Verification items for the finished model (mm, model axes). A direction names the side the tool comes from. Coordinates: 2 decimals unless noted, no trailing zeros. Write each loop counter-clockwise with the first axis right and the second up, starting at its lowest first coordinate (ties: lowest second). Pieces come first, ordered by that corner, then holes. Notation, with made-up numbers: (-35, 11.25) - (-30, 11.25) arc R21 ccw to (-30, 36.25) - close; hole circle Ø10 at (13.25, 25.5). An arc over 180 degrees is marked (long way). Use one line per item in the form item = value. Start each with the question number.
(1) Sectioned sample at A-A (z = 4.8). Record the cut outline in (x, y), and give its area (4 significant figures).
(2) Material ranges on line 1 (Z direction, x = 59.5, y = 18); line 2 (X direction, y = 38.5, z = 4.8); line 3 (Z direction, x = 56.7, y = 39.55), recorded low to high. Write a range as [from, to].
(3) Tool access check on faces 1 (the cylindrical face through (9.9, 11.3, -2.8)), 2 (the cylindrical face through (53.6, 39.53, 7.93)), 3 (the flat face through (44.376, -0.74, 59.833)). Record the directions out of +Z, -Z, +X, -X, +Y, -Y that give a thin tool (end or side, any length) a straight path to the whole face; none if there is none.
(4) Sectioned sample at D-D (z = 49). Record the cut outline in (x, y).
(5) Sectioned sample at B-B (y = 30.5). Record the cut outline in (x, z).
(6) Gauge pin test, flat ends, axial feed: pin 1 Ø2.5 at (x, z) = (58.5, 11.5) entering from +Y; pin 2 Ø4 at (x, y) = (52, 33) entering from -Z. Record the tip position at first contact, or that the pin passes through.
(7) Sectioned sample at C-C (z = 73.2). Count the separate pieces of the cut face and the enclosed holes in it, and give its area (3 significant figures).
(8) Mould release check, pull along Z, two halves, no side actions. Record for faces 4 (the flat face through (3, 37, 75)), 5 (the flat face through (-0.5, 42, 47.8)): released by +Z, released by -Z, zero draft, split by the parting line, or undercut.
from build123d import *

# Parameters (mm, degrees)
ESBO_O1_W                 = 63
ESBO_O1_H                 = 45
ESBO_O1_W_2               = 60
ESBO_O1_H_2               = 42
RESSALTO_EXTRUS_O2_DEPTH  = 1.5
RESSALTO_EXTRUS_O3_START  = 1.5
ESBO_O1_3_W               = 63
ESBO_O1_3_H               = 45
ESBO_O1_3_W_2             = 60
ESBO_O1_3_H_2             = 42
RESSALTO_EXTRUS_O3_DEPTH  = 75
RESSALTO_EXTRUS_O4_DEPTH  = 15
CORTE_EXTRUS_O1_DEPTH     = 27
ESBO_O4_W                 = 63
ESBO_O4_H                 = 45
RESSALTO_EXTRUS_O6_DEPTH  = 1.5
ESBO_O5_W                 = 63
ESBO_O5_H                 = 1.5
CORTE_EXTRUS_O2_DEPTH     = 109.436617432
RESSALTO_EXTRUS_O7_START  = 42
ESBO_O6_R                 = 1.3
RESSALTO_EXTRUS_O7_DEPTH  = 5
ESPELHAR2_START           = 42
ESPELHAR2_COPY_1_SKETCH_R = 1.3
ESPELHAR2_COPY_1_DEPTH    = 5
RESSALTO_EXTRUS_O8_START  = -5.5
RESSALTO_EXTRUS_O8_DEPTH  = 5.5
ESBO_O7_W                 = 3
ESBO_O7_H                 = 3
RESSALTO_EXTRUS_O9_DEPTH  = 25.5


with BuildPart() as part:
    # Esboço1 → Ressalto-extrusão2 (new body)
    # profile 1 of 3: a face of its own
    with BuildSketch(Plane.XY):
        with Locations((30, 21)):
            Rectangle(ESBO_O1_W, ESBO_O1_H)
        with Locations((30, 21)):
            Rectangle(ESBO_O1_W_2, ESBO_O1_H_2, mode=Mode.SUBTRACT)
    # profile 2 of 3: a face of its own
    with BuildSketch(Plane.XY):
        with Locations((30, 21)):
            Rectangle(ESBO_O1_W_2, ESBO_O1_H_2)
        with BuildLine():
            ThreePointArc((12.174114264, 11.987815308), (11.9, 11.3), (12.174114264, 10.612184692))
            Line((12.174114264, 10.612184692), (18.25, 4.2))
            Line((18.25, 4.2), (41.75, 4.2))
            Line((41.75, 4.2), (47.825885736, 10.612184692))
            ThreePointArc((47.825885736, 10.612184692), (48.1, 11.3), (47.825885736, 11.987815308))
            Line((47.825885736, 11.987815308), (41.75, 18.4))
            Line((41.75, 18.4), (18.25, 18.4))
            Line((18.25, 18.4), (12.174114264, 11.987815308))
        make_face(mode=Mode.SUBTRACT)
    # profile 3 of 3: a face of its own
    with BuildSketch(Plane.XY):
        with Locations((30, 21)):
            Rectangle(ESBO_O1_W_2, ESBO_O1_H_2)
        with BuildLine():
            ThreePointArc((10.722342792, 13.363445925), (9.9, 11.3), (10.722342792, 9.236554075))
            Line((10.722342792, 9.236554075), (17.389851698, 2.2))
            Line((17.389851698, 2.2), (42.610148302, 2.2))
            Line((42.610148302, 2.2), (49.277657208, 9.236554075))
            ThreePointArc((49.277657208, 9.236554075), (50.1, 11.3), (49.277657208, 13.363445925))
            Line((49.277657208, 13.363445925), (42.610148302, 20.4))
            Line((42.610148302, 20.4), (17.389851698, 20.4))
            Line((17.389851698, 20.4), (10.722342792, 13.363445925))
        make_face(mode=Mode.SUBTRACT)
    extrude(amount=RESSALTO_EXTRUS_O2_DEPTH)

    # Esboço1<3> → Ressalto-extrusão3 (add)
    with BuildSketch(Plane.XY.offset(RESSALTO_EXTRUS_O3_START)):
        with Locations((30, 21)):
            Rectangle(ESBO_O1_3_W, ESBO_O1_3_H)
        with Locations((30, 21)):
            Rectangle(ESBO_O1_3_W_2, ESBO_O1_3_H_2, mode=Mode.SUBTRACT)
    extrude(amount=RESSALTO_EXTRUS_O3_DEPTH)

    # Esboço2 → Ressalto-extrusão4 (add)
    with BuildSketch(Plane(origin=(0, 0, 0), x_dir=(1, 0, 0), z_dir=(0, 1, 0))):
        with BuildLine():
            Line((18.25, -54.8), (41.75, -54.8))
            Line((41.75, -54.8), (48.66440786, -62.248218844))
            ThreePointArc((48.66440786, -62.248218844), (49.654140055, -63.822712297), (50, -65.65))
            Line((50, -65.65), (51.5, -65.65))
            ThreePointArc((51.5, -65.65), (51.050382071, -63.274525986), (49.763730218, -61.227684497))
            Line((49.763730218, -61.227684497), (42.404219824, -53.3))
            Line((42.404219824, -53.3), (17.595780176, -53.3))
            Line((17.595780176, -53.3), (10.236269782, -61.227684497))
            ThreePointArc((10.236269782, -61.227684497), (8.949617929, -63.274525986), (8.5, -65.65))
            Line((8.5, -65.65), (10, -65.65))
            ThreePointArc((10, -65.65), (10.345859945, -63.822712297), (11.33559214, -62.248218844))
            Line((11.33559214, -62.248218844), (18.25, -54.8))
        make_face()
        with BuildLine():
            ThreePointArc((11.33559214, -69.051781156), (10.345859945, -67.477287703), (10, -65.65))
            Line((10, -65.65), (8.5, -65.65))
            ThreePointArc((8.5, -65.65), (8.949617929, -68.025474014), (10.236269782, -70.072315503))
            Line((10.236269782, -70.072315503), (16.2032846, -76.5))
            Line((16.2032846, -76.5), (18.25, -76.5))
            Line((18.25, -76.5), (11.33559214, -69.051781156))
        make_face()
        with BuildLine():
            Line((51.5, -65.65), (50, -65.65))
            ThreePointArc((50, -65.65), (49.654140055, -67.477287703), (48.66440786, -69.051781156))
            Line((48.66440786, -69.051781156), (41.75, -76.5))
            Line((41.75, -76.5), (43.7967154, -76.5))
            Line((43.7967154, -76.5), (49.763730218, -70.072315503))
            ThreePointArc((49.763730218, -70.072315503), (51.050382071, -68.025474014), (51.5, -65.65))
        make_face()
    extrude(amount=RESSALTO_EXTRUS_O4_DEPTH)

    # Esboço2<3> → Corte-extrusão1 (cut)
    with BuildSketch(Plane(origin=(0, 0, 0), x_dir=(1, 0, 0), z_dir=(0, 1, 0))):
        with BuildLine():
            Line((41.095780176, -56.3), (30, -56.3))
            Line((30, -56.3), (30, -75))
            Line((30, -75), (41.095780176, -75))
            Line((41.095780176, -75), (47.565085502, -68.031246809))
            ThreePointArc((47.565085502, -68.031246809), (48.5, -65.65), (47.565085502, -63.268753191))
            Line((47.565085502, -63.268753191), (41.095780176, -56.3))
        make_face()
        with BuildLine():
            Line((30, -75), (30, -56.3))
            Line((30, -56.3), (18.904219824, -56.3))
            Line((18.904219824, -56.3), (12.434914498, -63.268753191))
            ThreePointArc((12.434914498, -63.268753191), (11.5, -65.65), (12.434914498, -68.031246809))
            Line((12.434914498, -68.031246809), (18.904219824, -75))
            Line((18.904219824, -75), (30, -75))
        make_face()
    extrude(amount=-CORTE_EXTRUS_O1_DEPTH, mode=Mode.SUBTRACT)

    # Esboço4 → Ressalto-extrusão6 (add)
    with BuildSketch(Plane.XY.offset(76.5)):
        with Locations((30, 21)):
            Rectangle(ESBO_O4_W, ESBO_O4_H)
    extrude(amount=RESSALTO_EXTRUS_O6_DEPTH)

    # Esboço5 → Corte-extrusão2 (cut, through all)
    with BuildSketch(Plane.XY.offset(78)):
        with Locations((30, 42.75)):
            Rectangle(ESBO_O5_W, ESBO_O5_H)
    extrude(amount=-CORTE_EXTRUS_O2_DEPTH, mode=Mode.SUBTRACT)

    # Esboço6 → Ressalto-extrusão7 (add)
    with BuildSketch(Plane(origin=(0, 0, 0), x_dir=(1, 0, 0), z_dir=(0, 1, 0)).offset(RESSALTO_EXTRUS_O7_START)):
        with BuildLine():
            Line((60, -1.5), (60, -8.5))
            Line((60, -8.5), (55, -8.5))
            ThreePointArc((55, -8.5), (53.585786438, -7.914213562), (53, -6.5))
            Line((53, -6.5), (53, -1.5))
            Line((53, -1.5), (60, -1.5))
        make_face()
        with Locations(Location((56.7, -4.8, 0), (0, 0, 90))):
            Circle(ESBO_O6_R, mode=Mode.SUBTRACT)
    ressalto_extrus_o7 = extrude(amount=-RESSALTO_EXTRUS_O7_DEPTH)

    # Espelhar1: Ressalto-extrusão7 across plane
    add(ressalto_extrus_o7.mirror(Plane.XY.offset(39)))

    # Espelhar2: Ressalto-extrusão7 across plane
    add(ressalto_extrus_o7.mirror(Plane.ZY.offset(-30)))

    # Espelhar2 copy 1 sketch → Espelhar2 copy 1 (add)
    with BuildSketch(Plane(origin=(60, 0, 78), x_dir=(-1, 0, 0), z_dir=(0, 1, 0)).offset(ESPELHAR2_START)):
        with BuildLine():
            Line((60, -1.5), (60, -8.5))
            Line((60, -8.5), (55, -8.5))
            ThreePointArc((55, -8.5), (53.585786438, -7.914213562), (53, -6.5))
            Line((53, -6.5), (53, -1.5))
            Line((53, -1.5), (60, -1.5))
        make_face()
        with Locations(Location((56.7, -4.8, 0), (0, 0, 90))):
            Circle(ESPELHAR2_COPY_1_SKETCH_R, mode=Mode.SUBTRACT)
    extrude(amount=-ESPELHAR2_COPY_1_DEPTH)

    # Esboço1<4> → Ressalto-extrusão8 (add)
    with BuildSketch(Plane.XY.offset(RESSALTO_EXTRUS_O8_START)):
        with BuildLine():
            Line((17.389851698, 20.4), (10.722342792, 13.363445925))
            ThreePointArc((10.722342792, 13.363445925), (9.9, 11.3), (10.722342792, 9.236554075))
            Line((10.722342792, 9.236554075), (17.389851698, 2.2))
            Line((17.389851698, 2.2), (42.610148302, 2.2))
            Line((42.610148302, 2.2), (49.277657208, 9.236554075))
            ThreePointArc((49.277657208, 9.236554075), (50.1, 11.3), (49.277657208, 13.363445925))
            Line((49.277657208, 13.363445925), (42.610148302, 20.4))
            Line((42.610148302, 20.4), (17.389851698, 20.4))
        make_face()
        with BuildLine():
            ThreePointArc((12.174114264, 11.987815308), (11.9, 11.3), (12.174114264, 10.612184692))
            Line((12.174114264, 10.612184692), (18.25, 4.2))
            Line((18.25, 4.2), (41.75, 4.2))
            Line((41.75, 4.2), (47.825885736, 10.612184692))
            ThreePointArc((47.825885736, 10.612184692), (48.1, 11.3), (47.825885736, 11.987815308))
            Line((47.825885736, 11.987815308), (41.75, 18.4))
            Line((41.75, 18.4), (18.25, 18.4))
            Line((18.25, 18.4), (12.174114264, 11.987815308))
        make_face(mode=Mode.SUBTRACT)
    extrude(amount=RESSALTO_EXTRUS_O8_DEPTH)

    # Esboço7 → Ressalto-extrusão9 (add)
    with BuildSketch(Plane(origin=(0, 0, 0), x_dir=(1, 0, 0), z_dir=(0, 1, 0))):
        with Locations((58.5, -11.5)):
            Rectangle(ESBO_O7_W, ESBO_O7_H)
    ressalto_extrus_o9 = extrude(amount=RESSALTO_EXTRUS_O9_DEPTH)

    # Espelhar3: Ressalto-extrusão9 across plane
    add(ressalto_extrus_o9.mirror(Plane.ZY.offset(-30)))


solid = part.part
Answers below:
q1.outline = (-1.5, -1.5) - (61.5, -1.5) - (61.5, 42) - (58, 42) - (58, 37) - (60, 37) - (60, 0) - (0, 0) - (0, 37) - (2, 37) - (2, 42) - (-1.5, 42) - close; (4.6, 37) - (7, 37) - (7, 42) - (4.6, 42) - close; (53, 37) - (55.4, 37) - (55.4, 42) - (53, 42) - close
q1.area = 264.5 mm2
q2.line_1 = [0, 1.5], [10, 13], [76.5, 78]
q2.line_2 = [-1.5, 2], [4.6, 7], [53, 55.4], [58, 61.5]
q2.line_3 = [0, 3.5], [6.1, 8.5], [69.5, 71.9], [74.5, 78]
q3.face_1 = -Z, -X
q3.face_2 = +Y
q3.face_3 = +Y, -Y
q4.outline = (-1.5, -1.5) - (61.5, -1.5) - (61.5, 42) - (60, 42) - (60, 0) - (0, 0) - (0, 42) - (-1.5, 42) - close
q5.outline = (-1.5, 0) - (61.5, 0) - (61.5, 78) - (-1.5, 78) - close; hole (0, 1.5) - (60, 1.5) - (60, 76.5) - (0, 76.5) - close
q6.pin_1 = 25.5
q6.pin_2 = 0
q7.separate_pieces = 4
q7.enclosed_holes = 0
q7.area = 288 mm2
q8.face_4 = undercut
q8.face_5 = zero draft
